from build123d import *

# Parameters (mm, degrees)
SKETCH_W        = 14.75
SKETCH_H        = 14.75
PAD_DEPTH       = 12.5
SKETCH001_W     = 14.75
SKETCH001_H     = 12
POCKET_DEPTH    = 1.5
SKETCH002_W     = 1.375
SKETCH002_H     = 12
POCKET001_DEPTH = 2


with BuildPart() as part:
    # Sketch → Pad (new body)
    with BuildSketch(Plane.XY):
        with Locations((7.375, 7.375)):
            Rectangle(SKETCH_W, SKETCH_H)
    extrude(amount=PAD_DEPTH)

    # Sketch001 → Pocket (cut)
    with BuildSketch(Plane.XY.offset(12.5)):
        with Locations((7.375, 7.375)):
            Rectangle(SKETCH001_W, SKETCH001_H)
    extrude(amount=-POCKET_DEPTH, mode=Mode.SUBTRACT)

    # Sketch002 → Pocket001 (cut)
    with BuildSketch(Plane.XY.offset(11)):
        with Locations((0.6875, 7.375)):
            Rectangle(SKETCH002_W, SKETCH002_H)
        with Locations((14.0625, 7.375)):
            Rectangle(SKETCH002_W, SKETCH002_H)
    extrude(amount=-POCKET001_DEPTH, mode=Mode.SUBTRACT)


solid = part.part
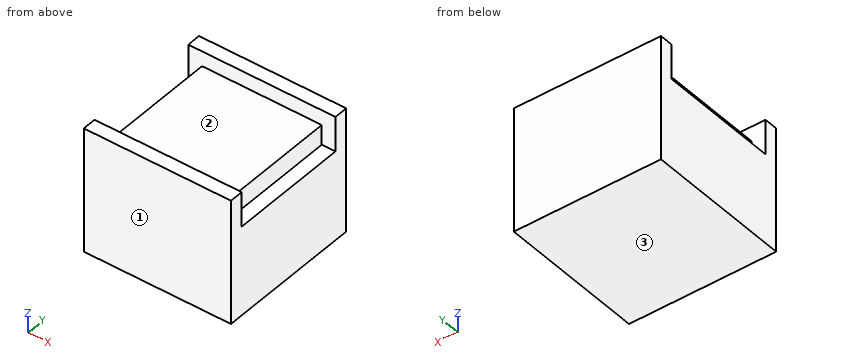
Could you check a few things on this model? Use its own coordinates, in mm. Face numbers are marked on the shaded views. Give positions to 0.01 mm unless a question says otherwise; leave off trailing zeros. Loops run counter-clockwise (first coordinate to the right, second up) from the corner with the lowest first, then second, coordinate; pieces in that order, holes last. Notation, with made-up numbers: (4, -26) -> (23, -26) arc R8 ccw to (23, -20) -> close; hole circle Ø4 at (6.5, 55). An arc over 180 degrees is marked (long way). Return JSON: item names as keys, results as strings.
Item 1: I need wall thicknesses on L1, parallel to Y at x = 13.75, z = 12.25 (3 decimals); L2, parallel to X at y = 5.5, z = 10 (3 decimals); L3, parallel to Z at x = 2, y = 2.25. Which ranges of each line are inside material? Lowest first, please. Write a range as from..to.
Geometry results:
{"L1": "y = 0..1.375, 13.375..14.75", "L2": "x = 1.375..13.375", "L3": "z = 0..11"}
Item 2: We'd pull the mould along Y, two halves only. Please class the marked faces 1, 2 and 3: +Y half, -Y half, draft (parallel to the pull), parting line (faces both ways), or undercut.
Geometry results:
{"face 1": "-Y half", "face 2": "undercut", "face 3": "draft"}
Item 3: I'm going to push flat-ended pins straight in: pin 1 (0.6 mm diameter, centred on y = 9.5, z = 10, fed in from +X) (3 decimals); pin 2 (2 mm diameter, centred on x = 12, y = 6, fed in from +Z). Where does each tip first touch, or does it pass through?
Geometry results:
{"pin 1": "stops at x = 13.375", "pin 2": "stops at z = 11"}
Item 4: If we section it at A-A on z = 11.5: List the corners of the cut face in (x, y) for me (3 decimals).
Geometry results:
{"outline": "(0, 0) -> (14.75, 0) -> (14.75, 1.375) -> (0, 1.375) -> close; (0, 13.375) -> (14.75, 13.375) -> (14.75, 14.75) -> (0, 14.75) -> close"}
Item 5: If we section it at C-C on y = 7.5: List the corners of the cut face in (x, z) for me (3 decimals), plus the area to 3 significant figures.
Geometry results:
{"outline": "(0, 0) -> (14.75, 0) -> (14.75, 9) -> (13.375, 9) -> (13.375, 11) -> (1.375, 11) -> (1.375, 9) -> (0, 9) -> close", "area": "157 mm²"}
Item 6: If we section it at B-B on x = 6: List the corners of the cut face in (y, z) for me (3 decimals), plus the area to 3 significant figures.
Geometry results:
{"outline": "(0, 0) -> (14.75, 0) -> (14.75, 12.5) -> (13.375, 12.5) -> (13.375, 11) -> (1.375, 11) -> (1.375, 12.5) -> (0, 12.5) -> close", "area": "166 mm²"}
Item 7: If we section it at D-D on z = 9.25: List the corners of the cut face in (x, y) for me (3 decimals), plus the area to 3 significant figures.
Geometry results:
{"outline": "(0, 0) -> (14.75, 0) -> (14.75, 1.375) -> (13.375, 1.375) -> (13.375, 13.375) -> (14.75, 13.375) -> (14.75, 14.75) -> (0, 14.75) -> (0, 13.375) -> (1.375, 13.375) -> (1.375, 1.375) -> (0, 1.375) -> close", "area": "185 mm²"}
